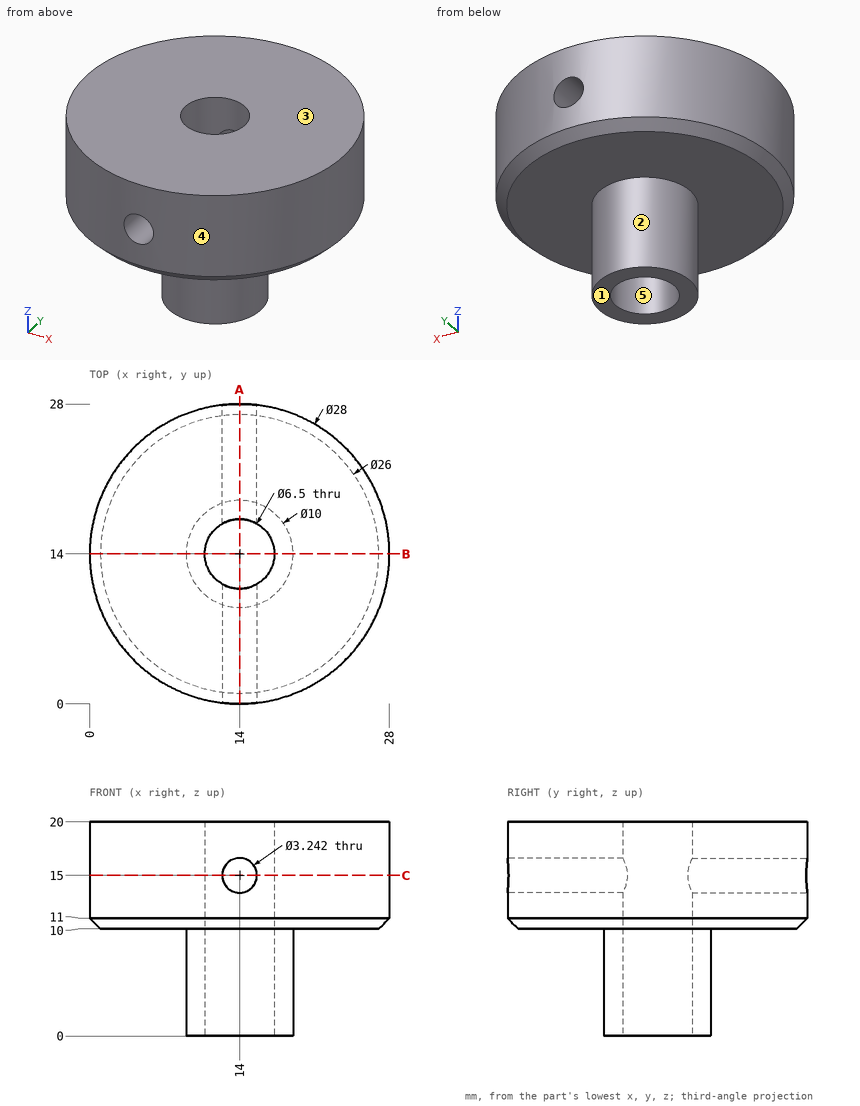
Design review of the part shown in the three views and the two pictorial views. Dimensions are in mm from the part's minimum x, y and z. A direction names the side the tool comes from. Coordinates: 2 decimals unless noted, no trailing zeros. Order: outer loops, then holes, each group sorted by start corner. A loop starts at its lowest first (then second) coordinate and runs counter-clockwise, first axis right, second up. Notation, with made-up numbers: (63, -12.75) - (119, -12.75) arc R18 ccw to (119, -8.75) - close; hole circle Ø2 at (-23, -33). An arc over 180 degrees is marked (long way). Answer as CSV lines item,"result". Start each with the question number.
1) Add section C-C (z = 15). State the section outline as (x, y) points.
2) Add section B-B (y = 14). State the section outline as (x, z) points.
3) To check wall thickness, follow line 1 along Z through (x, y) = (7.5, 6.25); line 2 along X through (y, z) = (25.5, 15); line 3 along X through (y, z) = (11.5, 6.75). State the ranges of each line that lie inside material, in increasing order. Write a range as [from, to].
4) Draft analysis for pull direction X (two halves, no side actions). For the marked faces 3, 4 and 5, state which applies: +X half, -X half, draft (parallel to the pull), parting line (faces both ways), or undercut.
5) Insertion check: P1, Ø1.5, axis at y = 10, z = 15.5, coming from the -X side; P2, Ø8.5, axis at x = 14, y = 14, coming from the +Z side; P3, Ø4, axis at x = 19, z = 13, coming from the -Y side; P4, Ø5, axis at y = 13.5, z = 6, coming from the +X side. Each pin has a flat end and moves straight along its axis. Give the tip position at first contact, or say it passes through.
6) Machinability: for the marked faces 1 and 2, which of the approach directions +Z, -Z, +X, -X, +Y, -Y give a long, thin tool a straight path to every point of the face, cutting with its end or side? Answer none if there is none.
7) Add section A-A (x = 14). State the section outline as (y, z) points.
Result:
1,outline,"(12.38, 0.09) - (12.38, 11.18) arc R3.25 cw to (12.38, 16.82) - (12.38, 27.91) arc R14 ccw to start; (15.62, 0.09) arc R14 ccw to (15.62, 27.91) - (15.62, 16.82) arc R3.25 cw to (15.62, 11.18) - close"
2,outline,"(0, 11) - (1, 10) - (9, 10) - (9, 0) - (10.75, 0) - (10.75, 20) - (0, 20) - close; (17.25, 0) - (19, 0) - (19, 10) - (27, 10) - (28, 11) - (28, 20) - (17.25, 20) - close"
3,line 1,"[10, 20]"
3,line 2,"[6.02, 12.38], [15.62, 21.98]"
3,line 3,"[9.67, 11.92], [16.08, 18.33]"
4,face 3,"draft"
4,face 4,"parting line"
4,face 5,"undercut"
5,P1,"x = 0.38"
5,P2,"z = 20"
5,P3,"y = 0.33"
5,P4,"x = 19"
6,face 1,"-Z, +X, -X, +Y, -Y"
6,face 2,"-Z"
7,outline,"(0, 11) - (1, 10) - (9, 10) - (9, 0) - (10.75, 0) - (10.75, 13.38) - (0, 13.38) - close; (0, 16.62) - (10.75, 16.62) - (10.75, 20) - (0, 20) - close; (17.25, 0) - (19, 0) - (19, 10) - (27, 10) - (28, 11) - (28, 13.38) - (17.25, 13.38) - close; (17.25, 16.62) - (28, 16.62) - (28, 20) - (17.25, 20) - close"
